Geometry: final body of the model. Coordinates: model frame, mm. Face numbers are marked on the shaded views. A direction names the side the tool comes from. Round coordinates to 2 decimals unless told otherwise and drop trailing zeros. Write each loop counter-clockwise with the first axis right and the second up, starting at its lowest first coordinate (ties: lowest second). Pieces come first, ordered by that corner, then holes. Notation, with made-up numbers: M 15,-32 L 48,-32 A17 cw 48,-8 Z; hole C 73.5,84.5 d2. An arc over 180 degrees is marked long. Use one line per item in the form item = value. Start each with the question number.
from build123d import *
from build123d.topology import SkipClean

# Parameters (mm, degrees)
SKETCH1_R           = 2.591205892
SKETCH1_R_2         = 1.143
BOSS_EXTRUDE4_DEPTH = 1.524
SKETCH5_R           = 6.1214
SKETCH5_R_2         = 4.7625
BOSS_EXTRUDE6_DEPTH = 5.8674
CUT_EXTRUDE1_START  = -6.1214001
CUT_EXTRUDE1_DEPTH  = 12.2428001


# Read off the part's stored shape, not the designer's step: Cut-Extrude1
with BuildPart() as part:
    # Sketch1 → Boss-Extrude4 (new body)
    with BuildSketch(Plane(origin=(0, 0, 0), x_dir=(1, 0, 0), z_dir=(0, 1, 0))):
        with BuildLine():
            ThreePointArc((6.273777289, 2.949269001), (9.7155, 0), (6.273777289, -2.949269001))
            ThreePointArc((6.273777289, -2.949269001), (5.577680109, -3.037502335), (5.034675871, -3.481892708))
            ThreePointArc((5.034675871, -3.481892708), (0, -6.1214), (-5.034675871, -3.481892708))
            ThreePointArc((-5.034675871, -3.481892708), (-5.577680109, -3.037502335), (-6.273777289, -2.949269001))
            ThreePointArc((-6.273777289, -2.949269001), (-9.7155, 0), (-6.273777289, 2.949269001))
            ThreePointArc((-6.273777289, 2.949269001), (-5.577680109, 3.037502335), (-5.034675871, 3.481892708))
            ThreePointArc((-5.034675871, 3.481892708), (0, 6.1214), (5.034675871, 3.481892708))
            ThreePointArc((5.034675871, 3.481892708), (5.577680109, 3.037502335), (6.273777289, 2.949269001))
        make_face()
        with Locations(Location((0, 0, 0), (0, 0, 90))):
            Circle(SKETCH1_R, mode=Mode.SUBTRACT)
        with Locations(Location((-6.731, 0, 0), (0, 0, 90))):
            Circle(SKETCH1_R_2, mode=Mode.SUBTRACT)
        with Locations(Location((6.731, 0, 0), (0, 0, 90))):
            Circle(SKETCH1_R_2, mode=Mode.SUBTRACT)
    extrude(amount=BOSS_EXTRUDE4_DEPTH)

    # Sketch5 → Boss-Extrude6 (add)
    with SkipClean():  # the faces are left unmerged after this step: merging them gives an invalid solid
        with BuildSketch(Plane(origin=(0, 1.524, 0), x_dir=(1, 0, 0), z_dir=(0, 1, 0))):
            with Locations(Location((0, 0, 0), (0, 0, 145.332951949))):
                Circle(SKETCH5_R)
            with Locations(Location((0, 0, 0), (0, 0, 90))):
                Circle(SKETCH5_R_2, mode=Mode.SUBTRACT)
        extrude(amount=BOSS_EXTRUDE6_DEPTH)

    # Cut-Extrude1 outline → Cut-Extrude1 (cut)
    with BuildSketch(Plane(origin=(0, 0, 0), x_dir=(0, 0, -1), z_dir=(1, 0, 0)).offset(CUT_EXTRUDE1_START)):
        with BuildLine():
            Line((-1.524, 3.846535004), (-1.524, 1.524))
            Line((-1.524, 1.524), (1.524, 1.524))
            Line((1.524, 1.524), (1.524, 3.846535004))
            ThreePointArc((1.524, 3.846535004), (1.545376148, 4.078566202), (1.608785003, 4.302786482))
            ThreePointArc((1.608785003, 4.302786482), (3.373151348, 6.540956309), (6.093287061, 7.3914))
            Line((6.093287061, 7.3914), (-6.093287061, 7.3914))
            ThreePointArc((-6.093287061, 7.3914), (-3.373151348, 6.540956309), (-1.608785003, 4.302786482))
            ThreePointArc((-1.608785003, 4.302786482), (-1.545376148, 4.078566202), (-1.524, 3.846535004))
        make_face()
    extrude(amount=CUT_EXTRUDE1_DEPTH, mode=Mode.SUBTRACT)


solid = part.part
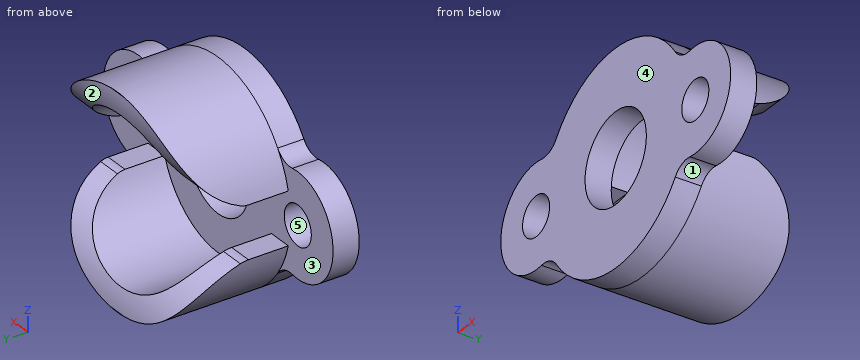
1. Ray query, probe 1 along X at (y, z) = (0.7, 0); probe 2 along Y at (x, z) = (8.25, -0.75); probe 3 along Z at (x, y) = (3, 2.5). Return the intervals inside material, ascending.
2. Contact query for flat-ended pins moving along their axis: pin 1 (1.6 mm diameter, centred on x = -5.5, y = 2.5, fed in from -Z); pin 2 (2 mm diameter, centred on x = -6.731, z = 0, fed in from +Y); pin 3 (1.5 mm diameter, centred on x = -5.5, y = 3, fed in from +Z); pin 4 (0.7 mm diameter, centred on x = -5, y = 3, fed in from +Z). Output: stop coordinate, or through.
3. Section query D-D (y = 1.25). Return loops of the section in (x, z), then the cut area to 3 significant figures.
4. Pull-direction query (X, two-part tool) for the marked faces 4 and 5; classes: released by +X, released by -X, zero draft, split by the parting line, or undercut.
5. Section query C-C (z = 0). Return loops of the section in (x, y), then the cut area to 3 significant figures.
6. Set-up query: the marked faces 1, 2 and 3. Return all of +Z, -Z, +X, -X, +Y, -Y with unobstructed straight access to the full face (end or side cutting, diameter ignored); none if empty.
7. Section query B-B (y = 2.75). Return loops of the section in (x, z) (1 decimal).
Checks:
q1.probe_1 = -9.72 to -7.87, -5.59 to -2.59, 2.59 to 5.59, 7.87 to 9.72
q1.probe_2 = 0 to 1.52
q1.probe_3 = -5.34 to -3.7, 3.7 to 5.34
q2.pin_1 = -3.92
q2.pin_2 = through
q2.pin_3 = 3.86
q2.pin_4 = 3.98
q3.outline = M -6.27,-2.95 A1.27 cw -5.03,-3.48 A6.12 ccw 5.03,-3.48 A1.27 cw 6.27,-2.95 A2.98 ccw long 6.27,2.95 A1.27 cw 5.03,3.48 A6.12 ccw -5.03,3.48 A1.27 cw -6.27,2.95 A2.98 ccw long Z; hole C -6.73,0 d2.29; hole C 0,0 d5.18; hole C 6.73,0 d2.29
q3.area = 127 mm^2
q4.face_4 = zero draft
q4.face_5 = undercut
q5.outline = M -9.72,0 L -7.87,0 L -7.87,1.52 L -9.72,1.52 Z; M -5.59,0 L -2.59,0 L -2.59,1.52 L -5.59,1.52 Z; M 2.59,0 L 5.59,0 L 5.59,1.52 L 2.59,1.52 Z; M 7.87,0 L 9.72,0 L 9.72,1.52 L 7.87,1.52 Z
q5.area = 14.7 mm^2
q6.face_1 = -Z, +Y, -Y
q6.face_2 = +X, -X, +Y
q6.face_3 = +Y
q7.outline = M -5.9,-1.5 A6.1 ccw 5.9,-1.5 L 4.5,-1.5 A4.8 cw -4.5,-1.5 Z; M -5.9,1.5 L -4.5,1.5 A4.8 cw 4.5,1.5 L 5.9,1.5 A6.1 ccw Z
